```python
from build123d import *

# Parameters (mm, degrees)
BOSS_EXTRUDE1_DEPTH = 46
CUT_EXTRUDE1_START  = -1
CUT_EXTRUDE1_DEPTH  = 44
CUT_EXTRUDE2_REACH  = 53.912


with BuildPart() as part:
    # Sketch1 → Boss-Extrude1 (new body)
    with BuildSketch(Plane(origin=(0, 0, 0), x_dir=(1, 0, 0), z_dir=(0, 1, 0))):
        Polygon((-19.895, 0), (19.895, 0), (19.895, 6), (6.5, 13.53), (-6.5, 13.53), (-19.895, 6), align=None)
    extrude(amount=BOSS_EXTRUDE1_DEPTH)

    # Sketch2 → Cut-Extrude1 (cut)
    with BuildSketch(Plane(origin=(0, 46, 0), x_dir=(1, 0, 0), z_dir=(0, 1, 0)).offset(CUT_EXTRUDE1_START)):
        Polygon((18.895, 5.414974095), (6.23819097, 12.53), (-6.23819097, 12.53), (-18.895, 5.414974095), (-18.895, 1), (18.895, 1), align=None)
    extrude(amount=-CUT_EXTRUDE1_DEPTH, mode=Mode.SUBTRACT)

    # Sketch3 → Cut-Extrude2 (cut, up to next)
    with BuildSketch(Plane.XZ, mode=Mode.PRIVATE) as cut_extrude2_sk1:
        with BuildLine():
            Line((-2.89, -9.97), (2.89, -9.97))
            ThreePointArc((2.89, -9.97), (4.17, -11.25), (2.89, -12.53))
            Line((2.89, -12.53), (-2.89, -12.53))
            ThreePointArc((-2.89, -12.53), (-4.17, -11.25), (-2.89, -9.97))
        make_face()
    cut_extrude2_tool1 = extrude(cut_extrude2_sk1.sketch, amount=-CUT_EXTRUDE2_REACH, mode=Mode.PRIVATE) & part.part
    add(cut_extrude2_tool1.solids().sort_by_distance((0, 0, -11.25))[0], mode=Mode.SUBTRACT)


solid = part.part
```
Model file for the job. Use its own axes, mm. A direction names the side the tool comes from. Give positions to 0.01 mm unless a question says otherwise; leave off trailing zeros. Order: outer loops, then holes, each group sorted by start corner. A loop starts at its lowest first (then second) coordinate and runs counter-clockwise, first axis right, second up.
1) Saw through at A-A, the plane z = -3.5. Write the cut outline in (x, y) (3 decimals), then the cut area to 3 significant figures.
2) Saw through at B-B, the plane y = 40.5. Write the cut outline in (x, z) (3 decimals).
3) Saw through at D-D, the plane z = -11.25. Write the cut outline in (x, y), then the cut area to 3 significant figures.
4) Saw through at C-C, the plane x = 11. Write the cut outline in (y, z), then the cut area to 3 significant figures.
5) 3-axis set-ups, long thin cutter, end or side, ignore diameter. For faces 5 (the cylindrical face through (4.17, 0.49, -11.22)), 6 (the flat face through (0, 22, -12.53)), 7 (the flat face through (0, 23, -13.53)): which of +Z, -Z, +X, -X, +Y, -Y reach the whole face in a straight line?
6) Wall check: probe 1 along X at (y, z) = (41.5, -2.5) (3 decimals); probe 2 along Y at (x, z) = (5.5, -10.5); probe 3 along Z at (x, y) = (2.5, 38.5). Give the ranges that are in metal, low to high.
7) Pin check, flat tips, straight feed: pin 1 (2 mm diameter, centred on y = 31.5, z = -11, fed in from +X); pin 2 (5 mm diameter, centred on x = 10.5, y = 23, fed in from -Z). Stop position of each tip, or through.
8) Mould opens along Y. For faces 1 (the flat face through (0, 46, -5)), 2 (the flat face through (18.895, 23, -3)), 3 (the flat face through (0, 0.5, -9.97)), 4 (the flat face through (-12.48, 23.31, -9.02)) say: +Y half, -Y half, draft (parallel to the pull), parting line (faces both ways), or undercut.
Computed:
1. outline: (-19.895, 0) - (19.895, 0) - (19.895, 46) - (-19.895, 46) - close; hole (-18.895, 1) - (18.895, 1) - (18.895, 45) - (-18.895, 45) - close
1. area: 168 mm2
2. outline: (-19.895, -6) - (-6.5, -13.53) - (6.5, -13.53) - (19.895, -6) - (19.895, 0) - (-19.895, 0) - close; hole (-18.895, -5.415) - (-6.238, -12.53) - (6.238, -12.53) - (18.895, -5.415) - (18.895, -1) - (-18.895, -1) - close
3. outline: (-10.56, 0) - (-4.17, 0) - (-4.17, 1) - (-8.52, 1) - (-8.52, 45) - (8.52, 45) - (8.52, 1) - (4.17, 1) - (4.17, 0) - (10.56, 0) - (10.56, 46) - (-10.56, 46) - close
3. area: 213 mm2
4. outline: (0, -11) - (46, -11) - (46, 0) - (0, 0) - close; hole (1, -9.85) - (45, -9.85) - (45, -1) - (1, -1) - close
4. area: 116 mm2
5. face 5: -Y
5. face 6: none
5. face 7: -Z, +X, -X, +Y, -Y
6. probe 1: x = -19.895 to -18.895, 18.895 to 19.895
6. probe 2: y = 0 to 1, 45 to 46
6. probe 3: z = -13.53 to -12.53, -1 to 0
7. pin 1: stops at x = 12.78
7. pin 2: stops at z = -12.69
8. face 1: +Y half
8. face 2: undercut
8. face 3: draft
8. face 4: undercut
